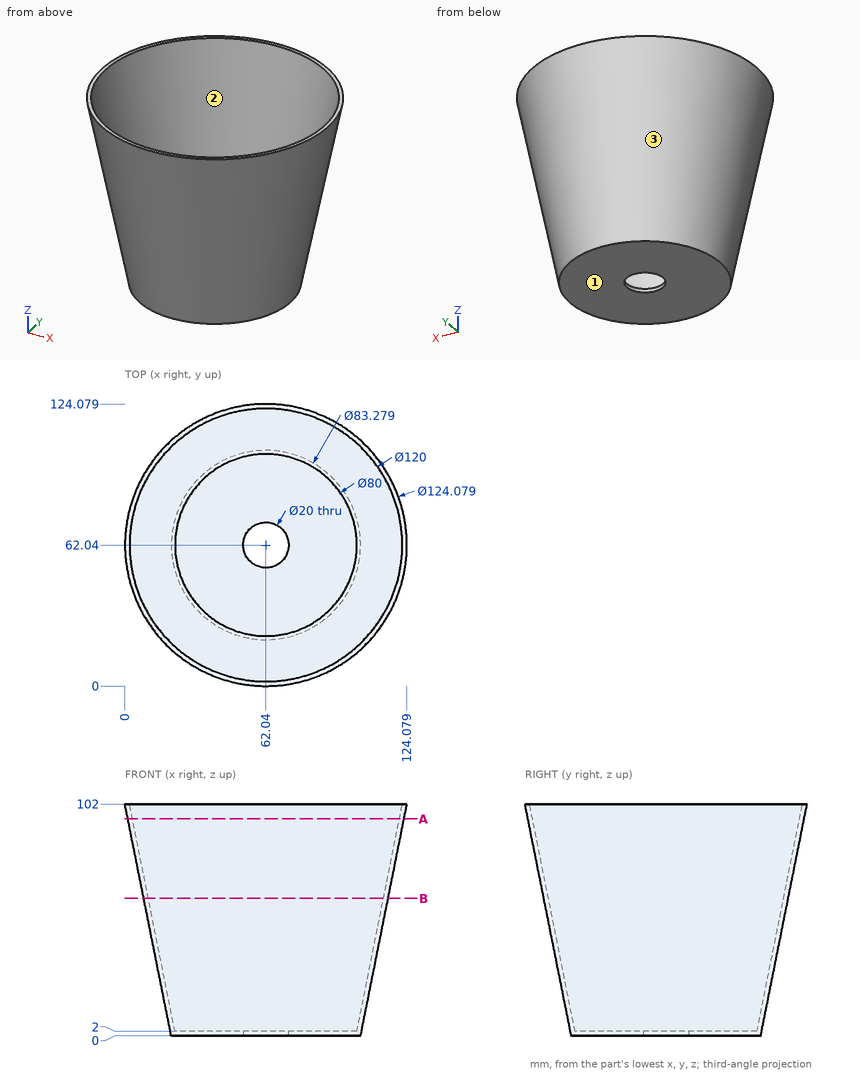
Here's the drawing with two shaded views (mm, measured from the low corner). I have some questions. Round coordinates to 2 decimals unless told otherwise and drop trailing zeros. Write each loop counter-clockwise with the first axis right and the second up, starting at its lowest first coordinate (ties: lowest second). Pieces come first, ordered by that corner, then holes.
(1) If I drill on probe 1 along Z at (x, y) = (43.5, 58); probe 2 along X at (y, z) = (94.5, 32) (1 decimal); probe 3 along Y at (x, z) = (49, 12) (1 decimal), over which ranges is the centre line in solid material (lowest first)?
Findings below:
probe 1: z = 0 to 2
probe 2: x = 26.6 to 29.4, 94.6 to 97.5
probe 3: y = 20 to 22.1, 102 to 104.1
(2) For pin 1 (4 mm diameter, centred on x = 34, z = 63.5, fed in from -Y) (1 decimal); pin 2 (3 mm diameter, centred on y = 24, z = 68, fed in from +X); pin 3 (10 mm diameter, centred on x = 43.5, y = 59, fed in from +Z), each with a flat end and sliding along its axis, tell me the tip position at first contact or that it passes through.
Findings below:
pin 1: stops at y = 14.3
pin 2: stops at x = 103.53
pin 3: stops at z = 2
(3) Thinking about a two-plate mould opening in Y: for the marked faces 1, 2 and 3, which applies, +Y half, -Y half, draft (parallel to the pull), parting line (faces both ways), or undercut?
Findings below:
face 1: draft
face 2: undercut
face 3: parting line
(4) Suppose I cut it at B-B on z = 60.5. Write out the boundary of the cut face in (x, y).
Findings below:
outline: circle Ø107.48 at (62.04, 62.04); hole circle Ø103.4 at (62.04, 62.04)
(5) Suppose I cut it at A-A on z = 95.5. Write out the boundary of the cut face in (x, y).
Findings below:
outline: circle Ø121.48 at (62.04, 62.04); hole circle Ø117.4 at (62.04, 62.04)
